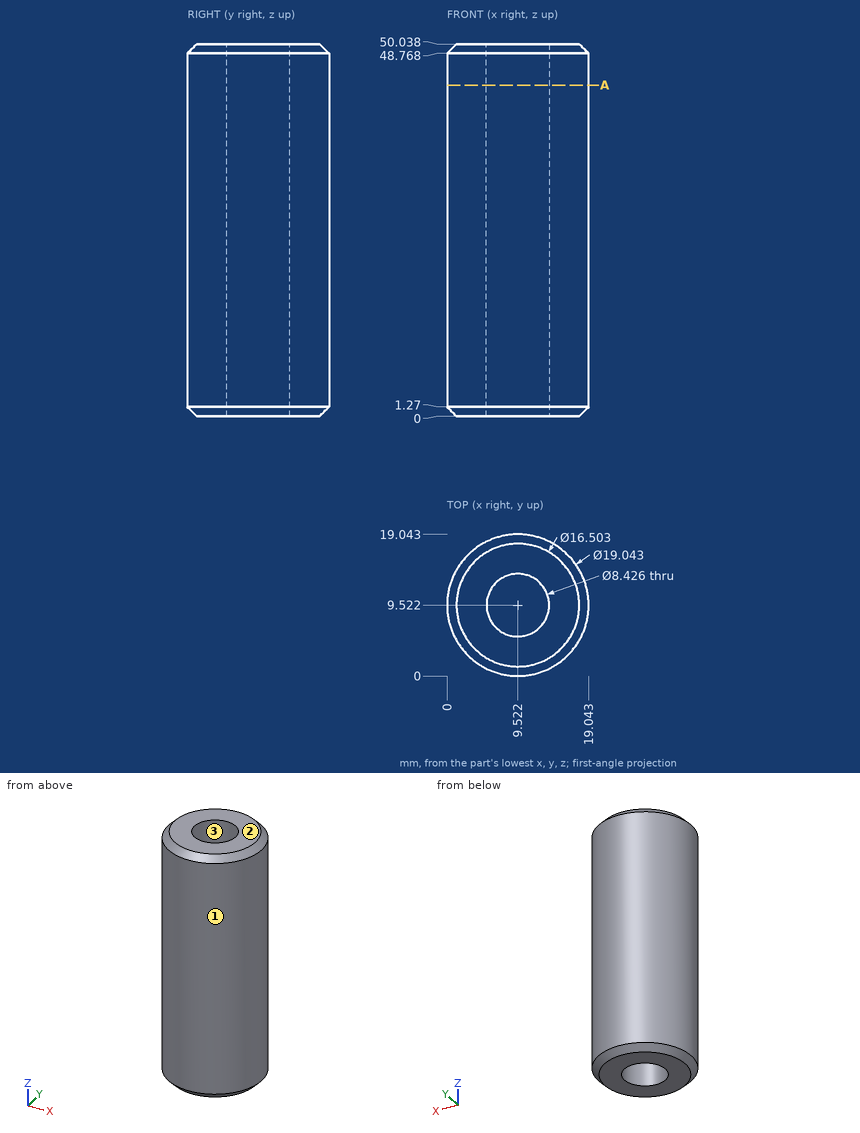
Can you work these out from the drawing? Everything is in mm from the part's minimum corner. Coordinates: 2 decimals unless noted, no trailing zeros. Loops run counter-clockwise (first coordinate to the right, second up) from the corner with the lowest first, then second, coordinate; pieces in that order, holes last. Notation, with made-up numbers: (-17, 36.5) - (8, 36.5) arc R10 cw to (8, 46.5) - close; hole circle Ø4 at (53, 52.5). An arc over 180 degrees is marked (long way). Answer as CSV lines item,"result".
Q1. If we section it at A-A, the plane z = 44.5: Write out the boundary of the cut face in (x, y) (1 decimal), and give its area (3 significant figures).
Response:
outline,"circle Ø19 at (9.5, 9.5); hole circle Ø8.4 at (9.5, 9.5)"
area,"229 mm2"
Q2. We'd pull the mould along Y, two halves only. Please class the marked faces 1, 2 and 3: pulls with the +Y half, pulls with the -Y half, needs draft (parallel to the pull), parting line crosses it, or undercut.
Response:
face 1,"parting line crosses it"
face 2,"needs draft"
face 3,"undercut"
Q3. If I drill on L1, parallel to Y at x = 12.25, z = 37.5 (1 decimal); L2, parallel to X at y = 12.75, z = 32 (1 decimal); L3, parallel to X at y = 11, z = 6 (1 decimal), over which ranges is the centre line in solid material (lowest first)? Write a range as [from, to].
Response:
L1,"[0.4, 6.3], [12.7, 18.6]"
L2,"[0.6, 6.8], [12.2, 18.5]"
L3,"[0.1, 5.6], [13.5, 18.9]"
Q4. For pin 1 (6 mm diameter, centred on x = 13.5, z = 6.5, fed in from -Y); pin 2 (2 mm diameter, centred on y = 11.5, z = 23, fed in from +X); pin 3 (8 mm diameter, centred on y = 3.5, z = 6, fed in from +X), each with a flat end and sliding along its axis, tell me the tip position at first contact or that it passes through.
Response:
pin 1,"y = 0.05"
pin 2,"x = 18.99"
pin 3,"x = 18.83"
